Could you check a few things on this model? Use its own coordinates, in mm. Face numbers are marked on the shaded views. A direction names the side the tool comes from. Coordinates: 2 decimals unless noted, no trailing zeros. Order: outer loops, then holes, each group sorted by start corner. A loop starts at its lowest first (then second) coordinate and runs counter-clockwise, first axis right, second up. Notation, with made-up numbers: (88, -11) - (146, -11) arc R31 ccw to (146, 22) - close; hole circle Ø10 at (6, 49). An arc over 180 degrees is marked (long way). Answer as a JSON object with one key per item and string values. Group by question number.
(1) Which directions (+Z, -Z, +X, -X, +Y, -Y) give clear straight access to the entire face, cutting with the end or side of a thin tool? Please do the marked faces 3, 4 and 5.
(2) Will these pins go through, and if not, where does the flat tip stop? P1, Ø0.5, axis at x = 0, y = -5.5, coming from the +Z side; P2, Ø1.5, axis at x = 1, y = -4.5, coming from the -Z side; P3, Ø0.7, axis at y = -8.5, z = 4.5, coming from the -X side; P4, Ø1, axis at y = -3, z = 0, coming from the +X side.
(3) We'd pull the mould along Z, two halves only. Please class the marked faces 1 and 2: pulls with the +Z half, pulls with the -Z half, needs draft (parallel to the pull), parting line crosses it, or undercut.
(4) Please list where these lines run through material, in increasing order: probe 1 along X at (y, z) = (-8.75, 4.25); probe 2 along Y at (x, z) = (0.5, 1.4); probe 3 along Y at (x, z) = (-0.1, 3.7).
(5) Imagine slicing it at C-C, the plane x = -0.5. Write out the boundary of the cut face in (y, z), and give its area (3 significant figures).
(6) Imagine slicing it at A-A, the plane z = 1.5. Write out the boundary of the cut face in (x, y).
(7) Imagine slicing it at B-B, the plane y = -6.5. Write out the boundary of the cut face in (x, z).
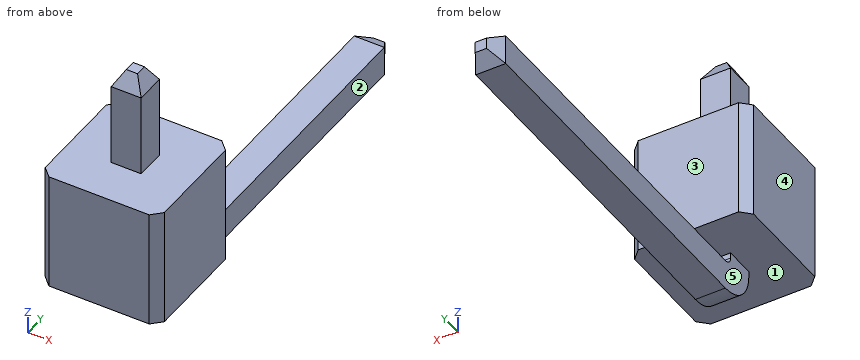
from build123d import *

# Parameters (mm, degrees)
SKETCH_2_W      = 0.64
SKETCH_2_H      = 0.64
CHAMFER_1_SIZE  = 0.2
CHAMFER_1_SIZE2 = 0.346410162
CHAMFER_2_SIZE  = 0.2
CHAMFER_2_SIZE2 = 0.346410162
SKETCH_3_W      = 2.54
SKETCH_3_H      = 2.54
EXTRUDE_1_DEPTH = 2.54
CHAMFER_3_SIZE  = 0.2


with BuildPart() as part:
    # По траектории1: sweep along a path in Эскиз1
    with BuildLine(Plane(origin=(0, 0, 0), x_dir=(0, 0, -1), z_dir=(1, 0, 0))) as sweep_1_path:
        Line((0, 0), (0, -8.04))
        ThreePointArc((0, -8.04), (-0.146446609, -8.393553391), (-0.5, -8.54))
        Line((-0.5, -8.54), (-5.27, -8.54))
    # Эскиз2 → По траектории1 (sweep)
    with BuildSketch(Plane(origin=(0, 0, 0), x_dir=(1, 0, 0), z_dir=(0, 1, 0))):
        Rectangle(SKETCH_2_W, SKETCH_2_H)
    sweep(path=sweep_1_path.line)

    # Фаска1
    chamfer_1_edges = [part.edges().sort_by_distance(p)[0] for p in [
        (0.32, -8.54, 5.27),
        (0, -8.86, 5.27),
        (-0.32, -8.54, 5.27),
        (0, -8.22, 5.27),
    ]]
    chamfer_1_side = [part.faces().sort_by_distance(p)[0] for p in [
        (0, -8.54, 5.27),
    ]]
    chamfer(chamfer_1_edges, length=CHAMFER_1_SIZE, length2=CHAMFER_1_SIZE2, reference=chamfer_1_side[0])

    # Фаска2
    chamfer_2_edges = [part.edges().sort_by_distance(p)[0] for p in [
        (0, 0, 0.32),
        (-0.32, 0, 0),
        (0, 0, -0.32),
        (0.32, 0, 0),
    ]]
    chamfer_2_side = [part.faces().sort_by_distance(p)[0] for p in [
        (0, 0, 0),
    ]]
    chamfer(chamfer_2_edges, length=CHAMFER_2_SIZE, length2=CHAMFER_2_SIZE2, reference=chamfer_2_side[0])

    # Эскиз3 → Бобышка-Вытянуть1 (add)
    with BuildSketch(Plane.XY.offset(0.62)):
        with Locations((0, -8.54)):
            Rectangle(SKETCH_3_W, SKETCH_3_H)
    extrude(amount=EXTRUDE_1_DEPTH)

    # Фаска3
    chamfer_3_edges = [part.edges().sort_by_distance(p)[0] for p in [
        (1.27, -9.81, 1.89),
        (1.27, -7.27, 1.89),
        (-1.27, -7.27, 1.89),
        (-1.27, -9.81, 1.89),
    ]]
    chamfer(chamfer_3_edges, length=CHAMFER_3_SIZE)


solid = part.part
Result set:
{
 "1": {"face 3": "+Z, +X, -X, +Y", "face 4": "+Z, -Z, -X, +Y, -Y", "face 5": "-Z, -X, +Y, -Y"},
 "2": {"P1": "stops at z = 0.32", "P2": "stops at z = -0.32", "P3": "stops at x = -0.32", "P4": "stops at x = 0.32"},
 "3": {"face 1": "undercut", "face 2": "needs draft"},
 "4": {"probe 1": "x = -0.32 to 0.32", "probe 2": "y = -9.81 to -7.27", "probe 3": "y = -8.86 to -8.22"},
 "5": {"outline": "(-9.81, 0.62) - (-7.27, 0.62) - (-7.27, 3.16) - (-9.81, 3.16) - close", "area": "6.45 mm^2"},
 "6": {"outline": "(-1.27, -9.61) - (-1.07, -9.81) - (1.07, -9.81) - (1.27, -9.61) - (1.27, -7.47) - (1.07, -7.27) - (-1.07, -7.27) - (-1.27, -7.47) - close"},
 "7": {"outline": "(-0.32, -0.32) - (0.32, -0.32) - (0.32, 0.32) - (-0.32, 0.32) - close"}
}
